from build123d import *

# Parameters (mm, degrees)
PAD012_DEPTH     = 5
SKETCH028_W      = 40
SKETCH028_H      = 3
POCKET005_DEPTH  = 5
POCKET007_DEPTH  = 2
HOLE_D           = 3.4
HOLE_DEPTH       = 25
HOLE_CBORE_D     = 6.1
HOLE_CBORE_DEPTH = 2.1


with BuildPart() as part:
    # Sketch017 → Pad012 (new body)
    with BuildSketch(Plane.XY):
        with BuildLine():
            Line((-125.019865, 68.987077), (125.0523, 68.987077))
            ThreePointArc((129.0523, 64.987077), (127.880727, 67.815504), (125.0523, 68.987077))
            Line((129.0523, 64.987077), (129.0523, -65.046829))
            ThreePointArc((125.0523, -69.046829), (127.880727, -67.875256), (129.0523, -65.046829))
            Line((125.0523, -69.046829), (-125.019865, -69.046829))
            ThreePointArc((-129.019865, -65.046829), (-127.848292, -67.875256), (-125.019865, -69.046829))
            Line((-129.019865, -65.046829), (-129.019865, 64.987077))
            ThreePointArc((-125.019865, 68.987077), (-127.848292, 67.815504), (-129.019865, 64.987077))
        make_face()
    extrude(amount=PAD012_DEPTH)

    # Sketch028 (on Face10 of Pad012) → Pocket005 (cut)
    with BuildSketch(Plane.XY.offset(5)):
        with Locations((-80.731997, 13.615229)):
            Rectangle(SKETCH028_W, SKETCH028_H)
        with Locations((-80.731997, 7.615229)):
            Rectangle(SKETCH028_W, SKETCH028_H)
        with Locations((-80.731997, 1.615229)):
            Rectangle(SKETCH028_W, SKETCH028_H)
        with Locations((-80.731997, -4.384771)):
            Rectangle(SKETCH028_W, SKETCH028_H)
        with Locations((-80.731997, -9.76974)):
            Rectangle(SKETCH028_W, SKETCH028_H)
        with Locations((-80.731997, -15.76974)):
            Rectangle(SKETCH028_W, SKETCH028_H)
    extrude(amount=-POCKET005_DEPTH, mode=Mode.SUBTRACT)

    # Sketch030 (on Face5 of Pocket005) → Pocket007 (cut)
    with BuildSketch(Plane.XY.offset(5)):
        with BuildLine():
            add(Edge.make_bspline(
                [(15.3717, 30.4705), (20.304277, 35.132774), (26.3615, 37.1956)],
                knots=[0, 0, 0, 1, 1, 1], degree=2))
            Line((26.3615, 37.1956), (26.3615, -31.859221))
            Line((26.3615, -31.859221), (29.97, -32.187271))
            Line((29.97, -32.187271), (29.97, 39.656))
            add(Edge.make_bspline(
                [(29.97, 39.656), (35.044575, 41.913307), (40.3036, 42.1163)],
                knots=[0, 0, 0, 1, 1, 1], degree=2))
            Line((40.3036, 42.1163), (40.3036, -48.0978))
            add(Edge.make_bspline(
                [(15.3717, -35.3038), (24.402502, -43.259792), (40.3036, -48.0978)],
                knots=[0, 0, 0, 1, 1, 1], degree=2))
            Line((15.3717, -35.3038), (15.3717, 30.4705))
        make_face()
        with BuildLine():
            add(Edge.make_bspline(
                [(45.3002, 44.0847), (51.3415, 45.0886), (55.7798, 44.794849)],
                knots=[0, 0, 0, 1, 1, 1], degree=2))
            Line((45.3002, 44.0847), (45.3002, -48.3978))
            add(Edge.make_bspline(
                [(45.3002, -48.3978), (50.487595, -49.138817), (55.7798, -48.5358)],
                knots=[0, 0, 0, 1, 1, 1], degree=2))
            Line((55.7798, -48.5358), (55.7798, 44.794849))
        make_face()
        with BuildLine():
            Line((58.0863, 44.3344), (58.0863, -6.569482))
            Line((58.0863, -6.569482), (72.830238, -6.569482))
            Line((72.830238, -6.569482), (72.830238, -30.86281))
            Line((72.830238, -30.86281), (69.074577, -30.715408))
            Line((69.074577, -30.715408), (69.074577, -10.083365))
            Line((69.074577, -10.083365), (58.1125, -10.083365))
            Line((58.1125, -10.083365), (58.1125, -47.3498))
            add(Edge.make_bspline(
                [(58.1125, -47.3498), (76.588104, -43.74934), (85.2152, -34.4005)],
                knots=[0, 0, 0, 1, 1, 1], degree=2))
            Line((85.2152, -34.4005), (85.2152, 3.085874))
            Line((85.2152, 3.085874), (68.937401, 3.085874))
            Line((68.937401, 3.085874), (68.937401, 28.534903))
            Line((68.937401, 28.534903), (69.012573, 28.534903))
            Line((69.012573, 28.534903), (72.55024, 28.534903))
            Line((72.55024, 28.534903), (72.55024, 7.45628))
            Line((72.55024, 7.45628), (85.1532, 7.45628))
            Line((85.1532, 7.45628), (85.1532, 31.1882))
            add(Edge.make_bspline(
                [(58.0863, 44.3344), (75.314171, 40.982338), (85.1532, 31.1882)],
                knots=[0, 0, 0, 1, 1, 1], degree=2))
        make_face()
    extrude(amount=-POCKET007_DEPTH, mode=Mode.SUBTRACT)

    # Hole
    with Locations(Plane.XY.offset(5)):
        with Locations((121.0523, 60.987077), (-121.019865, 60.987077), (-121.019865, -61.046829), (121.0523, -61.046829)):
            CounterBoreHole(HOLE_D / 2, HOLE_CBORE_D / 2, HOLE_CBORE_DEPTH, depth=HOLE_DEPTH)


with BuildPart() as part_1:
    # Body003 placement: moved
    add(part.part.moved(Location((0, 0, 110))))


solid = part_1.part
The model under review builds one solid part; all positions refer to its coordinate system, in mm. A direction names the side the tool comes from. Round coordinates to 2 decimals unless told otherwise and drop trailing zeros. Order: outer loops, then holes, each group sorted by start corner. A loop starts at its lowest first (then second) coordinate and runs counter-clockwise, first axis right, second up. Notation, with made-up numbers: (50, 28.25) -> (65, 28.25) arc R25 cw to (65, 59.25) -> close; hole circle Ø9 at (64.5, 64). An arc over 180 degrees is marked (long way). Use CSV: the item, a comma, the result in double quotes. Start each with the question number.
(1) Consider section C-C on z = 111. State how many separate pieces and enclosed holes the cut face has, and give its area (3 significant figures).
(2) Wall thickness on probe 1 along X at (y, z) = (4, 114.8); probe 2 along X at (y, z) = (-29, 113.35); probe 3 along X at (y, z) = (-10, 114.25): over which ranges is each line inside the solid? List them lowest first. Write a range as from..to.
(3) Mouldability with a two-part tool opening along X and no side actions: class faces 1 (the face through (2, -69.047, 112)), 2 (the face through (-119.612, 58.281, 113.965)), 3 (the face through (129.052, 1, 112)) as pulls with the +X half, pulls with the -X half, needs draft (parallel to the pull), parting line crosses it, or undercut.
(4) Insertion check: pin 1 (4 mm diameter, centred on x = 121.05, y = -61.05, fed in from +Z). The pin has a flat end and moves straight along its axis. Give the tip position at first contact, or say it passes through.
(5) Tool access review of faces 4 (the face through (-81, 12.115, 113)), 5 (the face through (123.87, -62.21, 113.96)), 6 (the face through (2, 1, 115)): name each direction out of +Z, -Z, +X, -X, +Y, -Y from which nothing blocks a thin tool from reaching the whole face with its end or side.
(6) Consider section B-B on y = 19. Write out the cut boundary in (x, z).
(7) Consider section A-A on x = -98. Write out the cut boundary in (y, z).
Responses:
1,separate pieces,"1"
1,enclosed holes,"10"
1,area,"34,900 mm²"
2,probe 1,"-129.02..15.37, 26.36..29.97, 40.3..45.3, 55.78..58.09, 68.94..129.05"
2,probe 2,"-129.02..15.37, 26.36..29.97, 40.3..45.3, 55.78..58.11, 69.07..72.83, 85.22..129.05"
2,probe 3,"-129.02..-100.73, -60.73..15.37, 26.36..29.97, 40.3..45.3, 55.78..72.83, 85.22..129.05"
3,face 1,"needs draft"
3,face 2,"undercut"
3,face 3,"pulls with the +X half"
4,pin 1,"z = 112.9"
5,face 4,"+Z, -Z"
5,face 5,"+Z"
5,face 6,"+Z, +X, -X, +Y, -Y"
6,outline,"(-129.02, 110) -> (129.05, 110) -> (129.05, 115) -> (85.15, 115) -> (85.15, 113) -> (72.55, 113) -> (72.55, 115) -> (68.94, 115) -> (68.94, 113) -> (58.09, 113) -> (58.09, 115) -> (55.78, 115) -> (55.78, 113) -> (45.3, 113) -> (45.3, 115) -> (40.3, 115) -> (40.3, 113) -> (29.97, 113) -> (29.97, 115) -> (26.36, 115) -> (26.36, 113) -> (15.37, 113) -> (15.37, 115) -> (-129.02, 115) -> close"
7,outline,"(-69.05, 110) -> (-17.27, 110) -> (-17.27, 115) -> (-69.05, 115) -> close; (-14.27, 110) -> (-11.27, 110) -> (-11.27, 115) -> (-14.27, 115) -> close; (-8.27, 110) -> (-5.88, 110) -> (-5.88, 115) -> (-8.27, 115) -> close; (-2.88, 110) -> (0.12, 110) -> (0.12, 115) -> (-2.88, 115) -> close; (3.12, 110) -> (6.12, 110) -> (6.12, 115) -> (3.12, 115) -> close; (9.12, 110) -> (12.12, 110) -> (12.12, 115) -> (9.12, 115) -> close; (15.12, 110) -> (68.99, 110) -> (68.99, 115) -> (15.12, 115) -> close"
